Part model, mm, in its own coordinate system. Coordinates: 2 decimals unless noted, no trailing zeros. Write each loop counter-clockwise with the first axis right and the second up, starting at its lowest first coordinate (ties: lowest second). Pieces come first, ordered by that corner, then holes. Notation, with made-up numbers: (61, 6) - (73, 6) arc R19 cw to (73, 22) - close; hole circle Ø6 at (24, -3.75). An arc over 180 degrees is marked (long way). Use one line per item in the form item = value. Start each with the question number.
Autodesk Inventor part; units mm, degrees
ref_plane "YZ Plane" through (0, 0, 0) normal (1, 0, 0) x (0, 1, 0)
ref_plane "XZ Plane" through (0, 0, 0) normal (0, 1, 0) x (-1, 0, 0)
ref_plane "XY Plane" through (0, 0, 0) normal (0, 0, 1) x (1, 0, 0)
sketch "Sketch1" plane through (0, 0, 0) normal (0, 0, 1) x (1, 0, 0)
  circle A0 centre (0, 0) radius 4.7625
  dimension "d0" = 9.525
extrude "Extrusion1" add sketch "Sketch1" along normal mid plane 25.4
sketch "Sketch3" plane through (0, 0, 12.7) normal (0, 0, 1) x (1, 0, 0)
  circle A0 centre (0, 0) radius 4.7625
hole "Hole1" at (0, 0, 12.7) direction (0, 0, -1) diameter 4.9784 end through all
sketch "Sketch4" plane through (0, 0, -12.7) normal (0, 0, -1) x (-1, 0, 0)
  circle A0 centre (0, 0) radius 3.175
  circle A1 centre (0, 0) radius 4.7625
  dimension "d10" = 6.35
extrude "Extrusion2" cut sketch "Sketch4" against normal blind 12.7
properties part number "EL2-008" material "Aluminum 6061"
Q1. Drill centre lines: probe 1 along Y at (x, z) = (0, -1.5) (3 decimals); probe 2 along Y at (x, z) = (0, 2); probe 3 along Z at (x, y) = (4, -2). Where is each one in solid material? Low to high.
Q2. Mould opens along Y. For faces 1 (the cylindrical face through (0.69, -3.1, -6.44)), 2 (the cylindrical face through (-0.748, -2.374, -0.178)), 3 (the flat face through (2, -2, 12.7)) say: released by +Y, released by -Y, zero draft, split by the parting line, or undercut.
Q3. Slice it at C-C (z = -1). List the corners of the cut face in (x, y) (3 decimals).
Q4. Slice it at D-D (y = -3.5). List the corners of the cut face in (x, z), plus the area to 3 significant figures.
Q5. Pin check, flat tips, straight feed: P1, Ø1, axis at x = 0.5, y = -1, coming from the +Z side; P2, Ø1.5, axis at y = 0, z = -9.5, coming from the +X side (3 decimals); P3, Ø4, axis at y = -3.5, z = -8, coming from the -X side. Stop position of each tip, or through.
Q6. Slice it at A-A (x = 0). List the corners of the cut face in (y, z) (1 decimal).
Solution:
q1.probe_1 = -3.175 to -2.489, 2.489 to 3.175
q1.probe_2 = -4.76 to -2.49, 2.49 to 4.76
q1.probe_3 = 0 to 12.7
q2.face_1 = split by the parting line
q2.face_2 = undercut
q2.face_3 = zero draft
q3.outline = circle Ø6.35 at (0, 0); hole circle Ø4.978 at (0, 0)
q4.outline = (-3.23, 0) - (3.23, 0) - (3.23, 12.7) - (-3.23, 12.7) - close
q4.area = 82.0 mm2
q5.P1 = through
q5.P2 = 3.175
q5.P3 = -2.8
q6.outline = (-4.8, 0) - (-3.2, 0) - (-3.2, -12.7) - (-2.5, -12.7) - (-2.5, 12.7) - (-4.8, 12.7) - close; (2.5, -12.7) - (3.2, -12.7) - (3.2, 0) - (4.8, 0) - (4.8, 12.7) - (2.5, 12.7) - close
